Source: CAD feature listing. Evaluate the final solid. Frame: model axes, mm. Face numbers are marked on the shaded views. Round coordinates to 2 decimals unless told otherwise and drop trailing zeros. Loops run counter-clockwise (first coordinate to the right, second up) from the corner with the lowest first, then second, coordinate; pieces in that order, holes last. Notation, with made-up numbers: (31, 2) -> (74, 2) arc R14 cw to (74, 19) -> close; hole circle Ø7 at (-31, -27). An arc over 180 degrees is marked (long way). Write item = value, one per line.
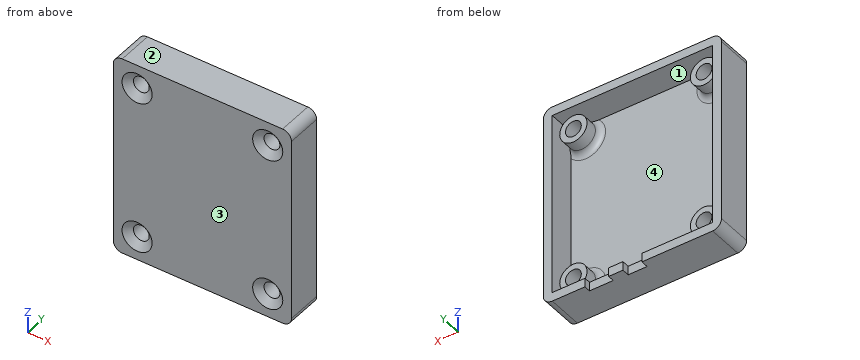
from build123d import *

# Parameters (mm, degrees)
SKETCH3_W                                           = 76.2
SKETCH3_H                                           = 86.36
BOSS_EXTRUDE2_DEPTH                                 = 15.24
SKETCH6_W                                           = 68.58
SKETCH6_H                                           = 78.74
CUT_EXTRUDE2_DEPTH                                  = 11.43
SKETCH7_R                                           = 5.842
SKETCH7_R_2                                         = 3.302
BOSS_EXTRUDE3_DEPTH                                 = 7.62
FILLET1_R                                           = 2.54
CSK_FOR_1_4_FLAT_HEAD_MACHINE_SCREW_100_D           = 6.7564
CSK_FOR_1_4_FLAT_HEAD_MACHINE_SCREW_100_DEPTH       = 91.44
CSK_FOR_1_4_FLAT_HEAD_MACHINE_SCREW_100_CSINK_D     = 12.8778
CSK_FOR_1_4_FLAT_HEAD_MACHINE_SCREW_100_CSINK_ANGLE = 100
CSK_FOR_1_4_FLAT_HEAD_MACHINE_SCREW_100_TIP         = 2.029827343
CUT_EXTRUDE4_REACH                                  = 118.176
SKETCH11_W                                          = 8.128
SKETCH11_H                                          = 3.175
CUT_EXTRUDE5_REACH                                  = 118.176
SKETCH12_W                                          = 10.16
SKETCH12_H                                          = 2.794
FILLET2_R                                           = 3.81


with BuildPart() as part:
    # Sketch3 → Boss-Extrude2 (new body)
    with BuildSketch(Plane(origin=(0, 0, 0), x_dir=(1, 0, 0), z_dir=(0, 1, 0))):
        with Locations((38.1, 43.18)):
            Rectangle(SKETCH3_W, SKETCH3_H)
    extrude(amount=BOSS_EXTRUDE2_DEPTH)

    # Sketch6 → Cut-Extrude2 (cut)
    with BuildSketch(Plane(origin=(0, 15.24, 0), x_dir=(1, 0, 0), z_dir=(0, 1, 0))):
        with Locations((38.1, 43.18)):
            Rectangle(SKETCH6_W, SKETCH6_H)
    extrude(amount=-CUT_EXTRUDE2_DEPTH, mode=Mode.SUBTRACT)

    # Sketch7 → Boss-Extrude3 (add)
    # profile 1 of 4: a face of its own
    with BuildSketch(Plane(origin=(0, 3.81, 0), x_dir=(1, 0, 0), z_dir=(0, 1, 0))):
        with Locations(Location((10.16, 76.2, 0), (0, 0, 90))):
            Circle(SKETCH7_R)
        with Locations(Location((10.16, 76.2, 0), (0, 0, 90))):
            Circle(SKETCH7_R_2, mode=Mode.SUBTRACT)
    # profile 2 of 4: a face of its own
    with BuildSketch(Plane(origin=(0, 3.81, 0), x_dir=(1, 0, 0), z_dir=(0, 1, 0))):
        with Locations(Location((66.04, 76.2, 0), (0, 0, 90))):
            Circle(SKETCH7_R)
        with Locations(Location((66.04, 76.2, 0), (0, 0, 90))):
            Circle(SKETCH7_R_2, mode=Mode.SUBTRACT)
    # profile 3 of 4: a face of its own
    with BuildSketch(Plane(origin=(0, 3.81, 0), x_dir=(1, 0, 0), z_dir=(0, 1, 0))):
        with Locations(Location((10.16, 10.16, 0), (0, 0, 90))):
            Circle(SKETCH7_R)
        with Locations(Location((10.16, 10.16, 0), (0, 0, 90))):
            Circle(SKETCH7_R_2, mode=Mode.SUBTRACT)
    # profile 4 of 4: a face of its own
    with BuildSketch(Plane(origin=(0, 3.81, 0), x_dir=(1, 0, 0), z_dir=(0, 1, 0))):
        with Locations(Location((66.04, 10.16, 0), (0, 0, 90))):
            Circle(SKETCH7_R)
        with Locations(Location((66.04, 10.16, 0), (0, 0, 90))):
            Circle(SKETCH7_R_2, mode=Mode.SUBTRACT)
    extrude(amount=BOSS_EXTRUDE3_DEPTH)

    # Fillet1
    # the kernel refuses this fillet: 2.54 mm, written as the material it adds along each edge
    with BuildSketch(Plane(origin=(10.16, 3.81, -76.2), x_dir=(0, 0, -1), z_dir=(1, 0, 0))) as fillet1_piece_1:
        with BuildLine():
            CenterArc((5.842 + FILLET1_R, FILLET1_R), FILLET1_R, 180, 90)
            Line((5.842, FILLET1_R), (5.842, 0))
            Line((5.842, 0), (5.842 + FILLET1_R, 0))
        make_face()
    revolve(axis=Axis((10.16, 3.81, -76.2), (0, 1, 0)))
    with BuildSketch(Plane(origin=(66.04, 3.81, -76.2), x_dir=(0, 0, -1), z_dir=(1, 0, 0))) as fillet1_piece_2:
        with BuildLine():
            CenterArc((5.842 + FILLET1_R, FILLET1_R), FILLET1_R, 180, 90)
            Line((5.842, FILLET1_R), (5.842, 0))
            Line((5.842, 0), (5.842 + FILLET1_R, 0))
        make_face()
    revolve(axis=Axis((66.04, 3.81, -76.2), (0, 1, 0)))
    with BuildSketch(Plane(origin=(10.16, 3.81, -10.16), x_dir=(0, 0, -1), z_dir=(1, 0, 0))) as fillet1_piece_3:
        with BuildLine():
            CenterArc((5.842 + FILLET1_R, FILLET1_R), FILLET1_R, 180, 90)
            Line((5.842, FILLET1_R), (5.842, 0))
            Line((5.842, 0), (5.842 + FILLET1_R, 0))
        make_face()
    revolve(axis=Axis((10.16, 3.81, -10.16), (0, 1, 0)))
    with BuildSketch(Plane(origin=(66.04, 3.81, -10.16), x_dir=(0, 0, -1), z_dir=(1, 0, 0))) as fillet1_piece_4:
        with BuildLine():
            CenterArc((5.842 + FILLET1_R, FILLET1_R), FILLET1_R, 180, 90)
            Line((5.842, FILLET1_R), (5.842, 0))
            Line((5.842, 0), (5.842 + FILLET1_R, 0))
        make_face()
    revolve(axis=Axis((66.04, 3.81, -10.16), (0, 1, 0)))

    # CSK for 1/4 Flat Head Machine Screw (100)1
    with Locations(Plane(origin=(0, 0, 0), x_dir=(-1, 0, 0), z_dir=(0, -1, 0))):
        with Locations((-10.16, 10.16), (-66.04, 10.16), (-66.04, 76.2), (-10.16, 76.2)):
            CounterSinkHole(CSK_FOR_1_4_FLAT_HEAD_MACHINE_SCREW_100_D / 2, CSK_FOR_1_4_FLAT_HEAD_MACHINE_SCREW_100_CSINK_D / 2, depth=CSK_FOR_1_4_FLAT_HEAD_MACHINE_SCREW_100_DEPTH, counter_sink_angle=CSK_FOR_1_4_FLAT_HEAD_MACHINE_SCREW_100_CSINK_ANGLE)
            with Locations((0, 0, -(CSK_FOR_1_4_FLAT_HEAD_MACHINE_SCREW_100_DEPTH + CSK_FOR_1_4_FLAT_HEAD_MACHINE_SCREW_100_TIP / 2))):  # 118° drill point
                Cone(0, CSK_FOR_1_4_FLAT_HEAD_MACHINE_SCREW_100_D / 2, CSK_FOR_1_4_FLAT_HEAD_MACHINE_SCREW_100_TIP, mode=Mode.SUBTRACT)

    # Sketch11 → Cut-Extrude4 (cut, up to next)
    with BuildSketch(Plane(origin=(0, 0, -86.36), x_dir=(-1, 0, 0), z_dir=(0, 0, -1)), mode=Mode.PRIVATE) as cut_extrude4_sk1:
        with Locations((-38.1, 13.6525)):
            Rectangle(SKETCH11_W, SKETCH11_H)
    cut_extrude4_tool1 = extrude(cut_extrude4_sk1.sketch, amount=-CUT_EXTRUDE4_REACH, mode=Mode.PRIVATE) & part.part
    add(cut_extrude4_tool1.solids().sort_by_distance((38.1, 13.6525, -86.36))[0], mode=Mode.SUBTRACT)

    # Sketch12 → Cut-Extrude5 (cut, up to next)
    with BuildSketch(Plane(origin=(0, 0, -86.36), x_dir=(-1, 0, 0), z_dir=(0, 0, -1)), mode=Mode.PRIVATE) as cut_extrude5_sk1:
        with Locations((-53.34, 13.843)):
            Rectangle(SKETCH12_W, SKETCH12_H)
    cut_extrude5_tool1 = extrude(cut_extrude5_sk1.sketch, amount=-CUT_EXTRUDE5_REACH, mode=Mode.PRIVATE) & part.part
    add(cut_extrude5_tool1.solids().sort_by_distance((53.34, 13.843, -86.36))[0], mode=Mode.SUBTRACT)

    # Fillet2
    fillet2_edges = [part.edges().sort_by_distance(p)[0] for p in [
        (0, 7.62, -86.36),
        (76.2, 7.62, -86.36),
        (76.2, 7.62, 0),
        (0, 7.62, 0),
    ]]
    fillet(fillet2_edges, radius=FILLET2_R)


solid = part.part
1. Section query A-A (y = 10). Give the number of separate pieces and of enclosed holes in the cut face, then the cut area to 3 significant figures.
Evaluation:
separate_pieces = 5
enclosed_holes = 5
area = 1,450 mm²
2. Line query: probe 1 along Z at (x, y) = (66.04, 7.75); probe 2 along X at (y, z) = (7.5, -76.2). Output: solid intervals per line, ascending. Write a range as from..to.
Evaluation:
probe_1 = -86.36..-82.55, -82.04..-79.58, -72.82..-70.36, -16..-13.54, -6.78..-4.32, -3.81..0
probe_2 = 0..3.81, 4.32..6.78, 13.54..16, 60.2..62.66, 69.42..71.88, 72.39..76.2
3. Contact query for flat-ended pins moving along their axis: pin 1 Ø1 at (x, z) = (72, -4.5) entering from +Y; pin 2 Ø1.4 at (y, z) = (14.5, -85.5) entering from -X; pin 3 Ø0.7 at (x, z) = (4.5, -4.5) entering from +Y; pin 4 Ø1.5 at (x, z) = (57.5, -33) entering from +Y. Output: stop coordinate, or through.
Evaluation:
pin_1 = 15.24
pin_2 = 0.74
pin_3 = 3.92
pin_4 = 3.81
4. Mould query, pull axis Z, two halves, no side actions, for the marked faces 1, 2, 3 and 4. Classes: released by +Z, released by -Z, zero draft, split by the parting line, or undercut.
Evaluation:
face_1 = undercut
face_2 = released by +Z
face_3 = zero draft
face_4 = undercut
5. Section query C-C (z = -41). Return the cut outline in (x, y).
Evaluation:
outline = (0, 0) -> (76.2, 0) -> (76.2, 15.24) -> (72.39, 15.24) -> (72.39, 3.81) -> (3.81, 3.81) -> (3.81, 15.24) -> (0, 15.24) -> close
